Check sheet for the modelled part. Datum: model origin and axes. Units: mm. A direction names the side the tool comes from. Round coordinates to 2 decimals unless told otherwise and drop trailing zeros. Loops run counter-clockwise (first coordinate to the right, second up) from the corner with the lowest first, then second, coordinate; pieces in that order, holes last. Notation, with made-up numbers: (69, -27.5) -> (100, -27.5) arc R7 ccw to (100, -16.5) -> close; hole circle Ø10 at (35.5, 24). An arc over 180 degrees is marked (long way). Use one line per item in the form item = value. Start each with the question number.
(1) Sectioned sample at A-A (y = -9). Record the cut outline in (x, z).
(2) Sectioned sample at B-B (x = -10.25). Record the cut outline in (y, z).
(3) Draft check along Z on faces 1 (the flat face through (6.986, 4.155, 11.457)), 2 (the flat face through (-0.105, 8.127, -11.457)), 3 (the cylindrical face through (14.985, 0.66, -30.986)), 4 (the flat face through (-7.09, 3.97, -11.46)). Enter one of: released by +Z, released by -Z, zero draft, split by the parting line, or undercut.
(4) Set-up check for faces 5 (the flat face through (0.105, -8.127, -11.457)), 6 (the flat face through (-6.986, -4.155, -11.457)), 7 (the flat face through (6.986, 4.155, -11.457)), 8 (the flat face through (7.09, -3.97, -11.46)): record each of +Z, -Z, +X, -X, +Y, -Y from which the full face is reachable in a straight line by a thin tool's end or side.
(5) Go/stop test with flat-tipped pins: pin 1 (10 mm diameter, centred on x = 1, y = 11, fed in from +Z); pin 2 (3 mm diameter, centred on y = 0, z = -25, fed in from +X); pin 3 (12 mm diameter, centred on x = -0.5, z = -4.5, fed in from -Y). Record where each tip stops, or that it passes through.
(6) Sectioned sample at C-C (z = 20). Record the cut outline in (x, y), and give its area (3 significant figures).
(7) Material ranges on probe 1 along Z at (x, y) = (10, 9.5); probe 2 along Z at (x, y) = (-5, 10.25); probe 3 along Z at (x, y) = (-0.5, -5), recorded low to high. Write a range as [from, to].
(8) Sectioned sample at D-D (x = -2). Record the cut outline in (y, z).
from build123d import *

# Parameters (mm, degrees)
BOSS_EXTRU_1_DEPTH = 30
BOSS_EXTRU_1_TAPER = 23
ESQUISSE2_R        = 15
BOSS_EXTRU_2_DEPTH = 2


with BuildPart() as part:
    # Esquisse1 → Boss.-Extru.1 (new body)
    with BuildSketch(Plane.XY):
        Polygon((15, 0), (7.5, 12.990381057), (-7.5, 12.990381057), (-15, 0), (-7.5, -12.990381057), (7.5, -12.990381057), align=None)
    boss_extru_1 = extrude(amount=BOSS_EXTRU_1_DEPTH, taper=BOSS_EXTRU_1_TAPER)

    # Symétrie1: Boss.-Extru.1 across plane
    add(boss_extru_1.mirror(Plane.XY))

    # Esquisse2 → Boss.-Extru.2 (add)
    with BuildSketch(Plane(origin=(0, 0, -30), x_dir=(-1, 0, 0), z_dir=(0, 0, -1))):
        Circle(ESQUISSE2_R)
    extrude(amount=BOSS_EXTRU_2_DEPTH)


solid = part.part
Checks:
q1.outline = (-12, -32) -> (12, -32) -> (12, -30) -> (-12, -30) -> close; (-9.8, 0) -> (-5.2, -9.4) -> (5.2, -9.4) -> (9.8, 0) -> (5.2, 9.4) -> (-5.2, 9.4) -> close
q2.outline = (-10.95, -32) -> (10.95, -32) -> (10.95, -30) -> (-10.95, -30) -> close; (-8.23, 0) -> (0, -9.69) -> (8.23, 0) -> (0, 9.69) -> close
q3.face_1 = released by +Z
q3.face_2 = undercut
q3.face_3 = zero draft
q3.face_4 = undercut
q4.face_5 = +X, -X, -Y
q4.face_6 = -X, -Y
q4.face_7 = +X, +Y
q4.face_8 = +X, -Y
q5.pin_1 = 16.47
q5.pin_2 = 3.48
q5.pin_3 = -12.99
q6.outline = (-5.2, 0) -> (-2.6, -4.5) -> (2.6, -4.5) -> (5.2, 0) -> (2.6, 4.5) -> (-2.6, 4.5) -> close
q6.area = 70.2 mm2
q7.probe_1 = [-32, -30]
q7.probe_2 = [-32, -30], [-6.46, 6.46]
q7.probe_3 = [-32, -30], [-18.82, 18.82]
q8.outline = (-14.87, -32) -> (14.87, -32) -> (14.87, -30) -> (-14.87, -30) -> close; (-12.99, 0) -> (-3.46, -22.44) -> (0, -26.52) -> (3.46, -22.44) -> (12.99, 0) -> (3.46, 22.44) -> (0, 26.52) -> (-3.46, 22.44) -> close
